Part model, mm, in its own coordinate system. Face numbers are marked on the shaded views. A direction names the side the tool comes from. Give positions to 0.01 mm unless a question says otherwise; leave off trailing zeros. Order: outer loops, then holes, each group sorted by start corner. A loop starts at its lowest first (then second) coordinate and runs counter-clockwise, first axis right, second up.
1. Slice it at A-A on x = -23.5. List the corners of the cut face in (y, z), and give its area (3 significant figures).
2. Slice it at B-B on y = 7. List the corners of the cut face in (x, z), and give its area (3 significant figures).
3. Drop flat-ended pins along their axis: pin 1 Ø12 at (x, y) = (-3, 2.5) entering from +Z; pin 2 Ø5 at (x, y) = (-1, -27) entering from +Z; pin 3 Ø1 at (y, z) = (17, 28.5) entering from +X. Give the stop position or say it passes through.
4. Probe line 1 (Y direction, x = -11, z = 4.5); line 2 (X direction, y = 13, z = 42.5); line 3 (Z direction, x = -22, y = 19). List the from-to ranges inside material, lowest first.
5. Slice it at D-D on x = 20. List the corners of the cut face in (y, z), and give its area (3 significant figures).
6. Slice it at C-C on z = 7.5. List the corners of the cut face in (x, y), and give its area (3 significant figures).
7. Which spindle directions (+Z, -Z, +X, -X, +Y, -Y) get a long thin tool onto all of the face, cutting with end or side? Do the marked faces 1 and 2. Say none if no direction does.
8. Mould opens along Y. For the marked faces 3, 4 and 5 say: +Y half, -Y half, draft (parallel to the pull), parting line (faces both ways), or undercut.
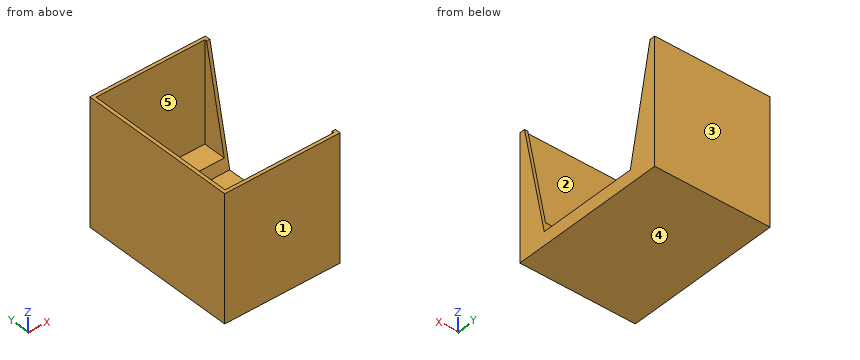
from build123d import *

# Parameters (mm, degrees)
F0_W     = 69
F0_H     = 94
F0_W_2   = 65
F0_H_2   = 90
F1_DEPTH = 60
F2_W     = 69
F2_H     = 94
F3_DEPTH = 15
F5_DEPTH = 40.4


with BuildPart() as f1:
    # F0 (on Top) → F1 (new body)
    with BuildSketch(Plane.XY):
        Rectangle(F0_W, F0_H)
        Rectangle(F0_W_2, F0_H_2, mode=Mode.SUBTRACT)
    extrude(amount=F1_DEPTH)

    # F2 (on face) → F3 (join)
    with BuildSketch(Plane(origin=(0, 0, 0), x_dir=(1, 0, 0), z_dir=(0, 0, -1))):
        Rectangle(F2_W, F2_H)
    extrude(amount=F3_DEPTH)

    # F4 (on face) → F5 (cut)
    with BuildSketch(Plane.YZ.offset(34.5)):
        Polygon((-30, -7), (0, -7), (30, -7), (45, 66), (0, 66), (-45, 66), align=None)
    extrude(amount=-F5_DEPTH, mode=Mode.SUBTRACT)


solid = f1.part
Data:
1. outline: (-47, -15) - (47, -15) - (47, 60) - (45, 60) - (45, 0) - (-45, 0) - (-45, 60) - (-47, 60) - close
1. area: 1,650 mm2
2. outline: (-34.5, -15) - (34.5, -15) - (34.5, -7) - (-5.9, -7) - (-5.9, 0) - (-32.5, 0) - (-32.5, 60) - (-34.5, 60) - close
2. area: 872 mm2
3. pin 1: stops at z = 0
3. pin 2: stops at z = -7
3. pin 3: stops at x = -32.5
4. line 1: y = -47 to -45, 45 to 47
4. line 2: x = -34.5 to -32.5
4. line 3: z = -15 to 0
5. outline: (-47, -15) - (47, -15) - (47, 60) - (45, 60) - (45, 0) - (31.44, 0) - (30, -7) - (-30, -7) - (-31.44, 0) - (-45, 0) - (-45, 60) - (-47, 60) - close
5. area: 1,220 mm2
6. outline: (-34.5, -47) - (34.5, -47) - (34.5, -32.98) - (32.5, -32.98) - (32.5, -45) - (-32.5, -45) - (-32.5, 45) - (32.5, 45) - (32.5, 32.98) - (34.5, 32.98) - (34.5, 47) - (-34.5, 47) - close
6. area: 504 mm2
7. face 1: +Z, -Z, +X, -X, -Y
7. face 2: +Z
8. face 3: +Y half
8. face 4: draft
8. face 5: undercut
